```python
from build123d import *

# Parameters (mm, degrees)
CYLINDER021_R     = 1
CYLINDER021_DEPTH = 50
ARRAY024_X_COUNT  = 2
ARRAY024_X_PITCH  = 8
CYLINDER022_R     = 1
CYLINDER022_DEPTH = 50
ARRAY025_Y_COUNT  = 2
ARRAY025_Y_PITCH  = 8
CYLINDER020_R     = 1
CYLINDER020_DEPTH = 10
ARRAY023_X_COUNT  = 2
ARRAY023_X_PITCH  = 12.5
ARRAY023_Y_COUNT  = 2
ARRAY023_Y_PITCH  = 21
CYLINDER019_R     = 1
CYLINDER019_DEPTH = 10
ARRAY022_X_COUNT  = 2
ARRAY022_X_PITCH  = 4
ARRAY022_Z_COUNT  = 2
ARRAY022_Z_PITCH  = 4
BOX016_W          = 8
BOX016_H          = 2
BOX016_DEPTH      = 8
ARRAY021_Y_COUNT  = 2
ARRAY021_Y_PITCH  = 4
BOX015_W          = 17
BOX015_H          = 25
BOX015_DEPTH      = 4


with BuildPart() as cameramountexpansionscrewshorizontal:
    # Cylinder021 → Cylinder021 (new body)
    with BuildSketch(Plane(origin=(-4, 12.5, 27), x_dir=(1, 0, 0), z_dir=(0, -1, 0))):
        Circle(CYLINDER021_R)
    extrude(amount=CYLINDER021_DEPTH)

    # Array024 X: CameraMountExpansionScrewsHorizontal ×2


with BuildPart() as cameramountexpansionscrewshorizontal_1:
    add(cameramountexpansionscrewshorizontal.part)
    with Locations(*[(i * ARRAY024_X_PITCH, 0, 0) for i in range(1, ARRAY024_X_COUNT)]):
        add(cameramountexpansionscrewshorizontal.part)


with BuildPart() as cameraexpansionscrews:
    # Cylinder022 → Cylinder022 (new body)
    with BuildSketch(Plane(origin=(-25, -4, 27), x_dir=(0, 0, -1), z_dir=(1, 0, 0))):
        Circle(CYLINDER022_R)
    extrude(amount=CYLINDER022_DEPTH)

    # Array025 Y: CameraExpansionScrews ×2


with BuildPart() as cameraexpansionscrews_1:
    add(cameraexpansionscrews.part)
    with Locations(*[(0, i * ARRAY025_Y_PITCH, 0) for i in range(1, ARRAY025_Y_COUNT)]):
        add(cameraexpansionscrews.part)

    # Fusion010: union CameraMountExpansionScrewsHorizontal
    add(cameramountexpansionscrewshorizontal_1.part)


with BuildPart() as camerascrews:
    # Cylinder020 → Cylinder020 (new body)
    with BuildSketch(Plane(origin=(-6.5, -10.5, 21), x_dir=(1, 0, 0), z_dir=(0, 0, 1))):
        Circle(CYLINDER020_R)
    extrude(amount=CYLINDER020_DEPTH)

    # Array023 X: CameraScrews ×2


with BuildPart() as camerascrews_1:
    add(camerascrews.part)
    with Locations(*[(i * ARRAY023_X_PITCH, 0, 0) for i in range(1, ARRAY023_X_COUNT)]):
        add(camerascrews.part)

    # Array023 Y: CameraScrews ×2


with BuildPart() as camerascrews_2:
    add(camerascrews_1.part)
    with Locations(*[(0, i * ARRAY023_Y_PITCH, 0) for i in range(1, ARRAY023_Y_COUNT)]):
        add(camerascrews_1.part)


with BuildPart() as cameramountplaneconnectorscrews:
    # Cylinder019 → Cylinder019 (new body)
    with BuildSketch(Plane(origin=(2, 5, 19), x_dir=(1, 0, 0), z_dir=(0, -1, 0))):
        Circle(CYLINDER019_R)
    extrude(amount=CYLINDER019_DEPTH)

    # Array022 X: CameraMountPlaneConnectorScrews ×2


with BuildPart() as cameramountplaneconnectorscrews_1:
    add(cameramountplaneconnectorscrews.part)
    with Locations(*[(-i * ARRAY022_X_PITCH, 0, 0) for i in range(1, ARRAY022_X_COUNT)]):
        add(cameramountplaneconnectorscrews.part)

    # Array022 Z: CameraMountPlaneConnectorScrews ×2


with BuildPart() as cameramountplaneconnectorscrews_2:
    add(cameramountplaneconnectorscrews_1.part)
    with Locations(*[(0, 0, i * ARRAY022_Z_PITCH) for i in range(1, ARRAY022_Z_COUNT)]):
        add(cameramountplaneconnectorscrews_1.part)


with BuildPart() as cameramountplaneconnector:
    # Box016 → Box016 (new body)
    with BuildSketch(Plane(origin=(-4, 1, 17), x_dir=(1, 0, 0), z_dir=(0, 0, 1))):
        with Locations((4, 1)):
            Rectangle(BOX016_W, BOX016_H)
    extrude(amount=BOX016_DEPTH)

    # Cut042: cut CameraMountPlaneConnectorScrews
    add(cameramountplaneconnectorscrews_2.part, mode=Mode.SUBTRACT)

    # Array021 Y: CameraMountPlaneConnector ×2


with BuildPart() as cameramountplaneconnector_1:
    add(cameramountplaneconnector.part)
    with Locations(*[(0, -i * ARRAY021_Y_PITCH, 0) for i in range(1, ARRAY021_Y_COUNT)]):
        add(cameramountplaneconnector.part)


with BuildPart() as cameramountplane3:
    # Box015 → Box015 (new body)
    with BuildSketch(Plane(origin=(-8.5, -12.5, 25), x_dir=(1, 0, 0), z_dir=(0, 0, 1))):
        with Locations((8.5, 12.5)):
            Rectangle(BOX015_W, BOX015_H)
    extrude(amount=BOX015_DEPTH)

    # Fusion009: union CameraMountPlaneConnector
    add(cameramountplaneconnector_1.part)

    # Cut043: cut CameraScrews
    add(camerascrews_2.part, mode=Mode.SUBTRACT)

    # Cut044: cut CameraExpansionScrews
    add(cameraexpansionscrews_1.part, mode=Mode.SUBTRACT)


solid = cameramountplane3.part
```
Design review of the part built by this model. Coordinates are the model's own, in mm. A direction names the side the tool comes from. Coordinates: 2 decimals unless noted, no trailing zeros. Order: outer loops, then holes, each group sorted by start corner. A loop starts at its lowest first (then second) coordinate and runs counter-clockwise, first axis right, second up. Notation, with made-up numbers: M 68.5,-7.5 L 99.5,-7.5 A24 cw 99.5,29.5 Z; hole C -21,72 d4. An arc over 180 degrees is marked long. Answer as a JSON object with one key per item and string values. Group by question number.
1) Mouldability with a two-part tool opening along Z and no side actions: class faces 5 (the flat face through (0, 2, 17)), 6 (the cylindrical face through (-7, 4, 28)), 7 (the flat face through (-8.5, 0, 27)) as pulls with the +Z half, pulls with the -Z half, needs draft (parallel to the pull), parting line crosses it, or undercut.
2) Wall thickness on L1, parallel to X at y = 1.55, z = 19; L2, parallel to Y at x = -2.5, z = 27; L3, parallel to Y at x = 0.25, z = 22: over which ranges is each line inside the solid? List them lowest first.
3) For pin 1 (1.6 mm diameter, centred on y = 4, z = 27, fed in from +X); pin 2 (3 mm diameter, centred on x = 2, z = 19, fed in from -Y); pin 3 (6 mm diameter, centred on y = 3, z = 21.5, fed in from -X); pin 4 (2.5 mm diameter, centred on x = -2, z = 23, fed in from +Y), all flat-tipped, find the tip position at first contact; note any pin that passes through.
4) Tool access review of faces 1 (the flat face through (0, -1, 21)), 2 (the flat face through (4, 2, 21)), 3 (the flat face through (-4, 2, 21)), 4 (the flat face through (0, 0, 29)): name each direction out of +Z, -Z, +X, -X, +Y, -Y from which nothing blocks a thin tool from reaching the whole face with its end or side.
5) Add section C-C, the plane z = 23. Write out the cut boundary in (x, y), then the cut area to 3 significant figures.
6) Add section B-B, the plane x = -2. Count the separate pieces of the cut face and the enclosed holes in it, then the cut area to 3 significant figures.
7) Add section A-A, the plane y = -10.5. Write out the cut boundary in (x, z), then the cut area to 3 significant figures.
8) Add section D-D, the plane x = 6. Write out the cut boundary in (y, z).
Computed values:
{
 "1": {"face 5": "pulls with the -Z half", "face 6": "undercut", "face 7": "needs draft"},
 "2": {"L1": "x = -4 to -3, -1 to 1, 3 to 4", "L2": "y = -12.5 to -5, -3 to 3, 5 to 12.5", "L3": "y = -3 to -1, 1 to 3"},
 "3": {"pin 1": "passes through", "pin 2": "stops at y = -3", "pin 3": "stops at x = -4", "pin 4": "stops at y = 3"},
 "4": {"face 1": "-Z, +X, -X", "face 2": "-Z, +X, +Y, -Y", "face 3": "-Z, -X, +Y, -Y", "face 4": "+Z, +X, -X, +Y, -Y"},
 "5": {"outline": "M -4,-3 L -3,-3 L -3,-1 L -4,-1 Z; M -4,1 L -3,1 L -3,3 L -4,3 Z; M -1,-3 L 1,-3 L 1,-1 L -1,-1 Z; M -1,1 L 1,1 L 1,3 L -1,3 Z; M 3,-3 L 4,-3 L 4,-1 L 3,-1 Z; M 3,1 L 4,1 L 4,3 L 3,3 Z", "area": "16.0 mm^2"},
 "6": {"separate pieces": "5", "enclosed holes": "2", "area": "110 mm^2"},
 "7": {"outline": "M -8.5,25 L -7.5,25 L -7.5,29 L -8.5,29 Z; M -5.5,25 L 5,25 L 5,29 L -5.5,29 Z; M 7,25 L 8.5,25 L 8.5,29 L 7,29 Z; hole C -4,27 d2; hole C 4,27 d2", "area": "45.7 mm^2"},
 "8": {"outline": "M -12.5,25 L -11.5,25 L -11.5,29 L -12.5,29 Z; M -9.5,25 L 9.5,25 L 9.5,29 L -9.5,29 Z; M 11.5,25 L 12.5,25 L 12.5,29 L 11.5,29 Z; hole C -4,27 d2; hole C 4,27 d2"}
}
